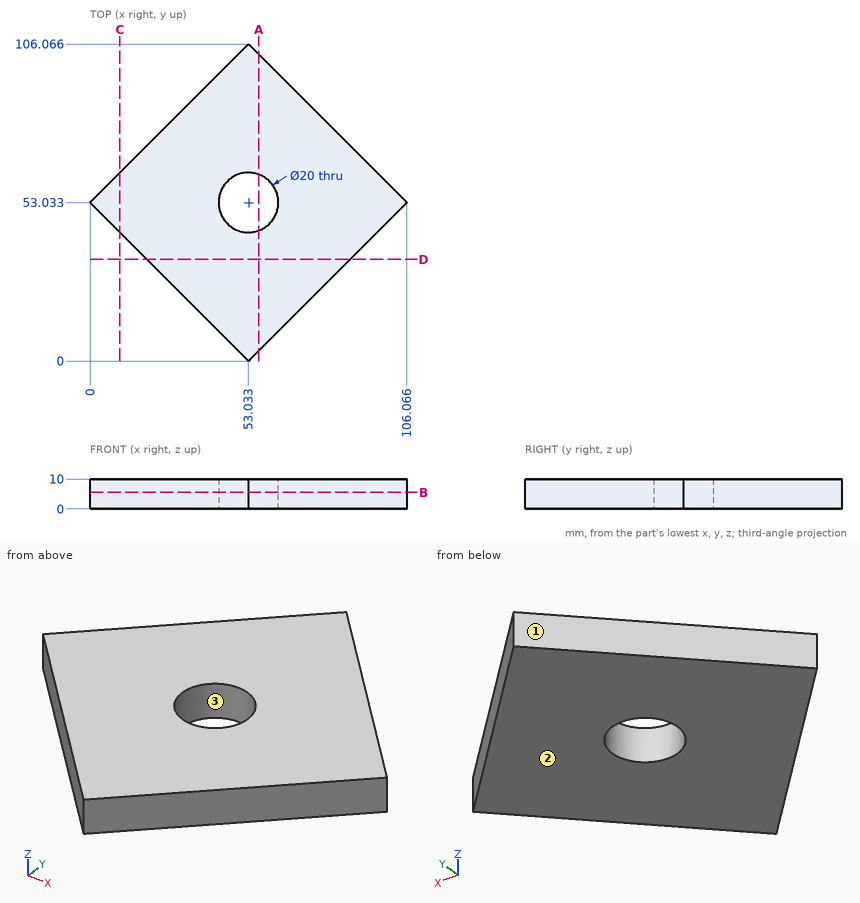
Geometry check sheet. Reference: drawing and pictorial views, mm from the part's lowest x, y, z. Round coordinates to 2 decimals unless told otherwise and drop trailing zeros. Loops run counter-clockwise (first coordinate to the right, second up) from the corner with the lowest first, then second, coordinate; pieces in that order, holes last. Notation, with made-up numbers: (61, -12) - (117, -12) arc R12 ccw to (117, 10) - close; hole circle Ø2 at (88.25, 45). An arc over 180 degrees is marked (long way). Answer in a Markdown table with one row per item. Add a question column.
Q1. Gauge pin test, flat ends, axial feed: pin 1 (8 mm diameter, centred on x = 75, y = 22.5, fed in from -Z); pin 2 (2 mm diameter, centred on x = 80, z = 9, fed in from -Y); pin 3 (16 mm diameter, centred on x = 53.03, y = 53.03, fed in from -Z); pin 4 (6 mm diameter, centred on y = 39, z = 7.5, fed in from +X). Record the tip position at first contact, or that the pin passes through.
Q2. Section check D-D on y = 34. Enter the section's corners in (x, z).
Q3. Material ranges on line 1 (Y direction, x = 59, z = 9); line 2 (Y direction, x = 56, z = 9.5); line 3 (X direction, y = 55, z = 8), recorded low to high.
Q4. Section check B-B on z = 5.5. Enter the section's corners in (x, y), plus the area to 3 significant figures.
Q5. Section check A-A on x = 56.5. Enter the section's corners in (y, z), plus the area to 3 significant figures.
Q6. Section check C-C on x = 10. Enter the section's corners in (y, z), plus the area to 3 significant figures.
Q7. Release check for a two-part mould opening along X. For the marked faces 1, 2 and 3 record: pulls with the +X half, pulls with the -X half, needs draft (parallel to the pull), parting line crosses it, or undercut.
Found:
| question | item | result |
|---|---|---|
| 1 | pin 1 | stops at z = 0 |
| 1 | pin 2 | stops at y = 25.97 |
| 1 | pin 3 | passes through |
| 1 | pin 4 | stops at x = 95.03 |
| 2 | outline | (19.03, 0) - (87.03, 0) - (87.03, 10) - (19.03, 10) - close |
| 3 | line 1 | y = 5.97 to 45.01, 61.06 to 100.1 |
| 3 | line 2 | y = 2.97 to 43.48, 62.58 to 103.1 |
| 3 | line 3 | x = 1.97 to 43.23, 62.84 to 104.1 |
| 4 | outline | (0, 53.03) - (53.03, 0) - (106.07, 53.03) - (53.03, 106.07) - close; hole circle Ø20 at (53.03, 53.03) |
| 4 | area | 5,310 mm² |
| 5 | outline | (3.47, 0) - (43.65, 0) - (43.65, 10) - (3.47, 10) - close; (62.41, 0) - (102.6, 0) - (102.6, 10) - (62.41, 10) - close |
| 5 | area | 804 mm² |
| 6 | outline | (43.03, 0) - (63.03, 0) - (63.03, 10) - (43.03, 10) - close |
| 6 | area | 200 mm² |
| 7 | face 1 | pulls with the -X half |
| 7 | face 2 | needs draft |
| 7 | face 3 | undercut |
